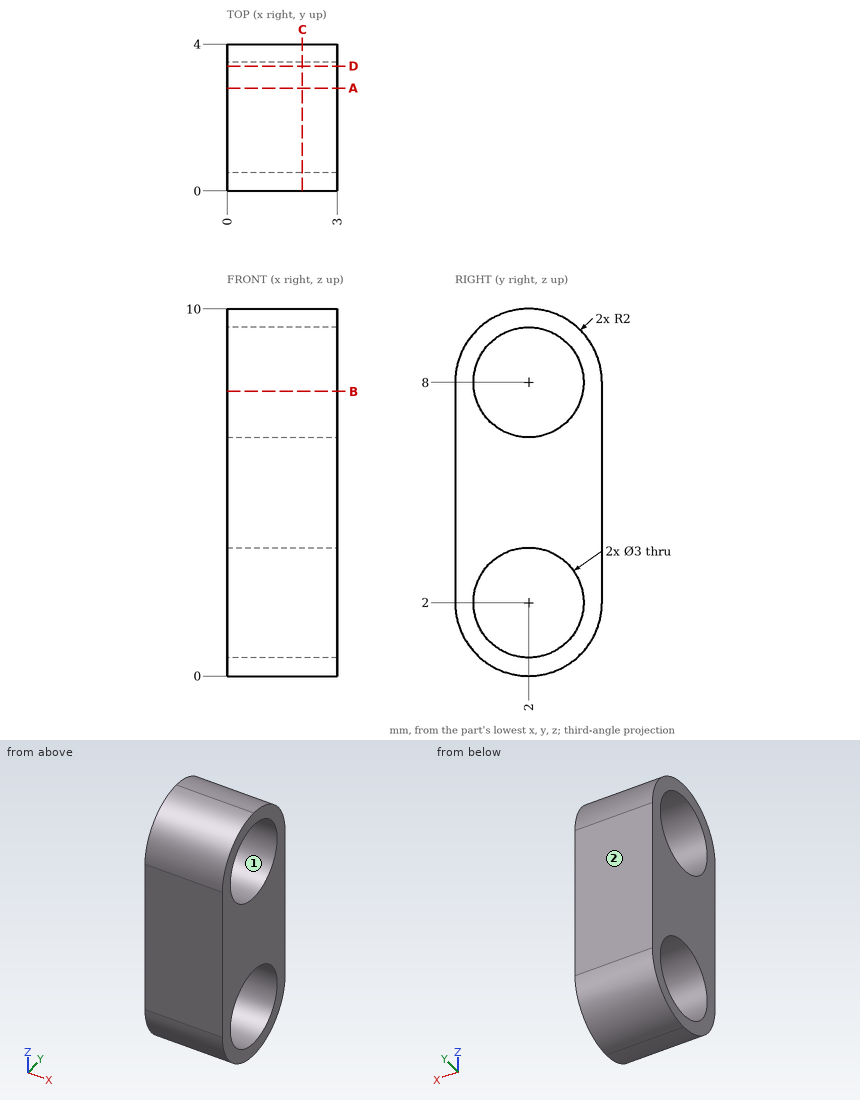
The figure shows three views and two pictorial views of one solid part (mm, origin at its lowest corner). Answer the questions. Round coordinates to 2 decimals unless told otherwise and drop trailing zeros. Order: outer loops, then holes, each group sorted by start corner. A loop starts at its lowest first (then second) coordinate and runs counter-clockwise, first axis right, second up. Notation, with made-up numbers: (37.25, 53) -> (48.25, 53) arc R23 ccw to (48.25, 92) -> close; hole circle Ø3 at (16, 38.5). An arc over 180 degrees is marked (long way). One line per item, written item: value.
Item 1: Find section C-C, the plane x = 2.05. Give the vertices of the cut face in (y, z).
Taken from the geometry:
outline: (0, 2) arc R2 ccw to (4, 2) -> (4, 8) arc R2 ccw to (0, 8) -> close; hole circle Ø3 at (2, 2); hole circle Ø3 at (2, 8)
Item 2: For a pull along Z with two mould halves and no side action, classify the marked faces 1 and 2 as released by +Z, released by -Z, zero draft, split by the parting line, or undercut.
Taken from the geometry:
face 1: undercut
face 2: zero draft
Item 3: Find section B-B, the plane z = 7.75. Give the vertices of the cut face in (x, y).
Taken from the geometry:
outline: (0, 0) -> (3, 0) -> (3, 0.52) -> (0, 0.52) -> close; (0, 3.48) -> (3, 3.48) -> (3, 4) -> (0, 4) -> close
Item 4: Straight lines are drawn through the part: L1, parallel to Z at x = 2.15, y = 3; L2, parallel to Y at x = 2.2, z = 2; L3, parallel to Z at x = 1, y = 0.9. For each, find the intervals that lie inside material, in ascending order.
Taken from the geometry:
L1: z = 0.27 to 0.88, 3.12 to 6.88, 9.12 to 9.73
L2: y = 0 to 0.5, 3.5 to 4
L3: z = 0.33 to 0.98, 3.02 to 6.98, 9.02 to 9.67
Item 5: Find section D-D, the plane y = 3.4. Give the vertices of the cut face in (x, z).
Taken from the geometry:
outline: (0, 0.57) -> (3, 0.57) -> (3, 1.46) -> (0, 1.46) -> close; (0, 2.54) -> (3, 2.54) -> (3, 7.46) -> (0, 7.46) -> close; (0, 8.54) -> (3, 8.54) -> (3, 9.43) -> (0, 9.43) -> close
Item 6: Find section A-A, the plane y = 2.8. Give the vertices of the cut face in (x, z), then the cut area to 3 significant figures.
Taken from the geometry:
outline: (0, 0.17) -> (3, 0.17) -> (3, 0.73) -> (0, 0.73) -> close; (0, 3.27) -> (3, 3.27) -> (3, 6.73) -> (0, 6.73) -> close; (0, 9.27) -> (3, 9.27) -> (3, 9.83) -> (0, 9.83) -> close
area: 13.8 mm2
